Geometry check sheet. Reference: drawing and pictorial views, mm from the part's lowest x, y, z. Coordinates: 2 decimals unless noted, no trailing zeros. Loops run counter-clockwise (first coordinate to the right, second up) from the corner with the lowest first, then second, coordinate; pieces in that order, holes last. Notation, with made-up numbers: (49, 54.25) - (55, 54.25) arc R20 ccw to (55, 73.25) - close; hole circle Ø9 at (-37.75, 17.5). An arc over 180 degrees is marked (long way). Use a Markdown table: item, result. Add a question column.
1) Sectioned sample at A-A, the plane x = 6.4. Enter the section's corners in (y, z), then the cut area to 3 significant figures.
2) Go/stop test with a flat-tipped pin: P1, Ø2, axis at y = 3, z = 10, coming from the -X side. Record where the tip stops, or that it passes through.
3) Draft check along X on the marked faces 1, 2, 3 and 4. Enter one of: pulls with the +X half, pulls with the -X half, needs draft (parallel to the pull), parting line crosses it, or undercut.
4) Sectioned sample at B-B, the plane y = 3.5. Enter the section's corners in (x, z), then the cut area to 3 significant figures.
5) Sectioned sample at C-C, the plane x = 25.4. Enter the section's corners in (y, z).
6) Thickness scan on line 1 (Z direction, x = 25.5, y = 1); line 2 (X direction, y = 5.5, z = 15) (1 decimal); line 3 (X direction, y = 6, z = 14.5) (1 decimal). Record the ranges inside material, lowest first.
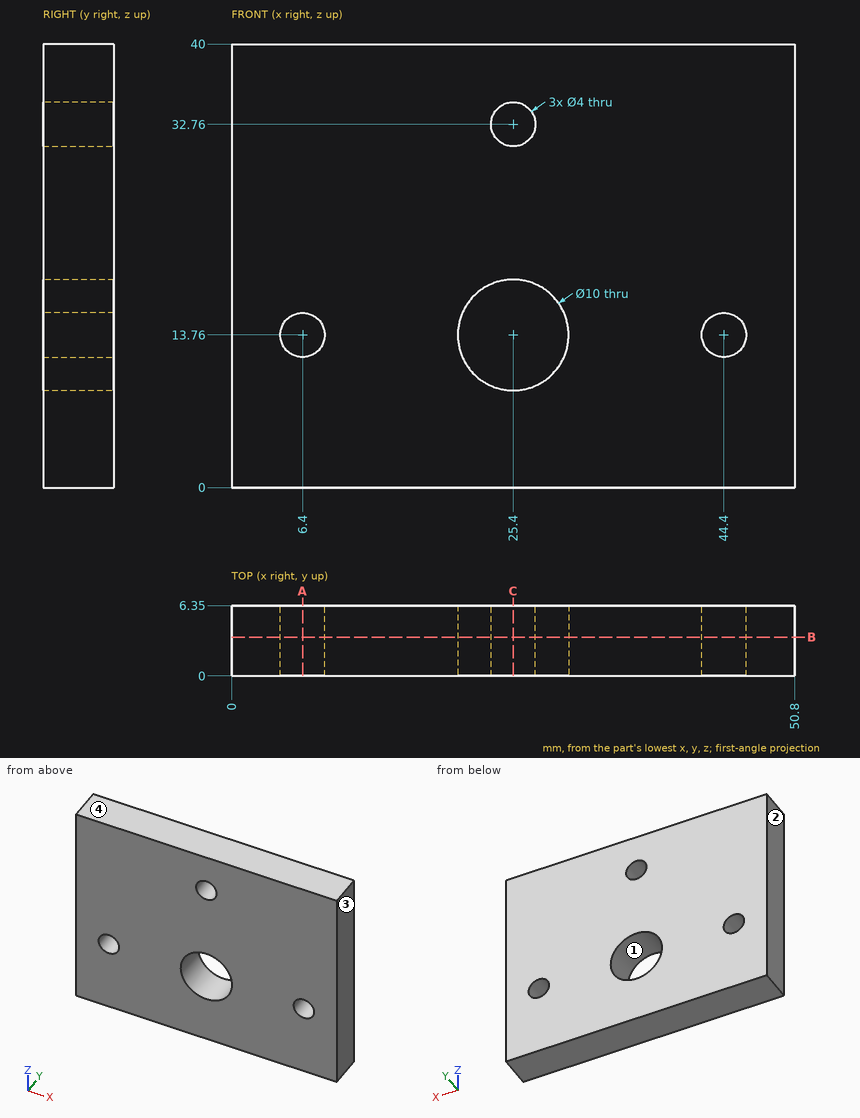
Solved:
| question | item | result |
|---|---|---|
| 1 | outline | (0, 0) - (6.35, 0) - (6.35, 11.76) - (0, 11.76) - close; (0, 15.76) - (6.35, 15.76) - (6.35, 40) - (0, 40) - close |
| 1 | area | 229 mm2 |
| 2 | P1 | stops at x = 0 |
| 3 | face 1 | undercut |
| 3 | face 2 | pulls with the -X half |
| 3 | face 3 | pulls with the +X half |
| 3 | face 4 | needs draft |
| 4 | outline | (0, 0) - (50.8, 0) - (50.8, 40) - (0, 40) - close; hole circle Ø4 at (6.4, 13.76); hole circle Ø10 at (25.4, 13.76); hole circle Ø4 at (25.4, 32.76); hole circle Ø4 at (44.4, 13.76) |
| 4 | area | 1,920 mm2 |
| 5 | outline | (0, 0) - (6.35, 0) - (6.35, 8.76) - (0, 8.76) - close; (0, 18.76) - (6.35, 18.76) - (6.35, 30.76) - (0, 30.76) - close; (0, 34.76) - (6.35, 34.76) - (6.35, 40) - (0, 40) - close |
| 6 | line 1 | z = 0 to 8.76, 18.76 to 30.76, 34.76 to 40 |
| 6 | line 2 | x = 0 to 4.8, 8 to 20.6, 30.2 to 42.8, 46 to 50.8 |
| 6 | line 3 | x = 0 to 4.5, 8.3 to 20.5, 30.3 to 42.5, 46.3 to 50.8 |
